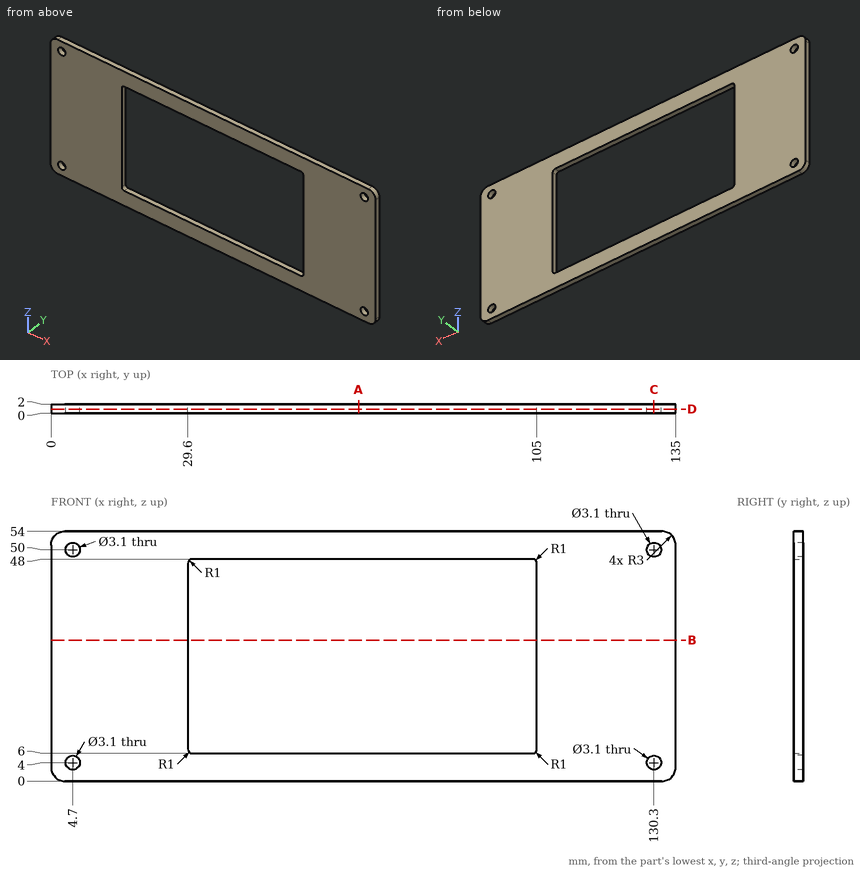
Could you check a few things on this drawing? It's one solid part, dimensions in mm from its lowest x, y, z. Give positions to 0.01 mm unless a question says otherwise; leave off trailing zeros. Write each loop counter-clockwise with the first axis right and the second up, starting at its lowest first coordinate (ties: lowest second). Pieces come first, ordered by that corner, then holes. Notation, with made-up numbers: M -31,29.25 L 8,29.25 A30 cw 8,64.25 Z; hole C 10.5,2 d1. An arc over 180 degrees is marked long. Put each result on its own line as item: value. Start each with the question number.
Item 1: If we section it at A-A, the plane x = 66.5: Write out the boundary of the cut face in (y, z), then the cut area to 3 significant figures.
Item 2: If we section it at B-B, the plane z = 30.5: Write out the boundary of the cut face in (x, y), then the cut area to 3 significant figures.
Item 3: I need wall thicknesses on L1, parallel to X at y = 1.1, z = 50; L2, parallel to X at y = 1.3, z = 19; L3, parallel to Z at x = 95, y = 1.5. Which ranges of each line are inside material? Lowest first, please. Write a range as from..to.
Item 4: If we section it at D-D, the plane y = 0.9: Write out the boundary of the cut face in (x, z).
Item 5: If we section it at C-C, the plane x = 130.3: Write out the boundary of the cut face in (y, z).
Values:
1. outline: M 0,0 L 2,0 L 2,6 L 0,6 Z; M 0,48 L 2,48 L 2,54 L 0,54 Z
1. area: 24.0 mm²
2. outline: M 0,0 L 29.6,0 L 29.6,2 L 0,2 Z; M 105,0 L 135,0 L 135,2 L 105,2 Z
2. area: 119 mm²
3. L1: 0..3.15, 6.25..128.75, 131.85..135
3. L2: 0..29.6, 105..135
3. L3: 0..6, 48..54
4. outline: M 0,3 A3 ccw 3,0 L 132,0 A3 ccw 135,3 L 135,51 A3 ccw 132,54 L 3,54 A3 ccw 0,51 Z; hole C 4.7,4 d3.1; hole C 4.7,50 d3.1; hole M 29.6,7 A1 ccw 30.6,6 L 104,6 A1 ccw 105,7 L 105,47 A1 ccw 104,48 L 30.6,48 A1 ccw 29.6,47 Z; hole C 130.3,4 d3.1; hole C 130.3,50 d3.1
5. outline: M 0,0 L 2,0 L 2,2.45 L 0,2.45 Z; M 0,5.55 L 2,5.55 L 2,48.45 L 0,48.45 Z; M 0,51.55 L 2,51.55 L 2,54 L 0,54 Z
